Geometry check sheet. Reference: the model listing, model coordinates, mm. A direction names the side the tool comes from. Coordinates: 2 decimals unless noted, no trailing zeros. Order: outer loops, then holes, each group sorted by start corner. A loop starts at its lowest first (then second) coordinate and runs counter-clockwise, first axis right, second up. Notation, with made-up numbers: (82, 27.25) - (135, 27.25) arc R20 cw to (135, 35.25) - close; hole circle Ø7 at (46.5, 37). An arc over 180 degrees is marked (long way). Return JSON: item names as keys, results as strings. Group by question number.
Item 1: Section check C-C on y = 31. Enter the section's corners in (x, z), then the cut area to 3 significant figures.
Item 2: Scan lines: probe 1 along Z at (x, y) = (13.5, 37); probe 2 along Y at (x, z) = (9, -0.5); probe 3 along X at (y, z) = (0.75, -12.5). Record each from-to range of solid material in increasing order.
Item 3: Gauge pin test, flat ends, axial feed: pin 1 (7.5 mm diameter, centred on x = 10.5, y = 15, fed in from -Z); pin 2 (0.6 mm diameter, centred on y = 0.5, z = -24, fed in from -X); pin 3 (2 mm diameter, centred on y = 27.5, z = -10, fed in from -X). Record the tip position at first contact, or that the pin passes through.
Item 4: Section check D-D on x = 13.5. Enter the section's corners in (y, z), then the cut area to 3 significant figures.
Item 5: Section check A-A on x = 24. Enter the section's corners in (y, z).
Item 6: Draft check along Z on faces 5 (the flat face through (25.2, 12.4, -25)), 6 (the cylindrical face through (16, 40.9, -11.4)), 7 (the flat face through (17.9, 2, -9.5)). Enter one of: pulls with the +Z half, pulls with the -Z half, needs draft (parallel to the pull), parting line crosses it, or undercut.
Item 7: Section check B-B on z = -11.5. Enter the section's corners in (x, y), then the cut area to 3 significant figures.
Item 8: Tool access check on faces 1 (the flat face through (11.5, 41, -12)), 2 (the cylindrical face through (7.518, 31.014, -17.871)), 3 (the cylindrical face through (16.56, 1.01, -16.92)), 4 (the flat face through (13, 16, 0)). Record the directions out of +Z, -Z, +X, -X, +Y, -Y that give a thin tool (end or side, any length) a straight path to the whole face; none if there is none.
from build123d import *

# Parameters (mm, degrees)
SKETCH1_W           = 25
SKETCH1_H           = 2
EXTRUDE_THIN1_DEPTH = 25
SKETCH2_R           = 6.0005
CUT_EXTRUDE1_DEPTH  = 36.411862419
BOSS_EXTRUDE1_DEPTH = 32
BOSS_EXTRUDE2_DEPTH = 2
SKETCH7_R           = 3.5
BOSS_EXTRUDE3_DEPTH = 18


with BuildPart() as part:
    # Sketch1 → Extrude-Thin1 (new body)
    with BuildSketch(Plane.XY):
        with Locations((12.5, 1)):
            Rectangle(SKETCH1_W, SKETCH1_H)
    extrude(amount=-EXTRUDE_THIN1_DEPTH)

    # Sketch2 → Cut-Extrude1 (cut, through all)
    with BuildSketch(Plane(origin=(0, 2, 0), x_dir=(1, 0, 0), z_dir=(0, 1, 0))):
        with BuildLine():
            ThreePointArc((3.839745962, 7.5), (3.839745962, 17.5), (12.5, 22.5))
            Line((12.5, 22.5), (12.5, 25))
            Line((12.5, 25), (0, 25))
            Line((0, 25), (0, 7.5))
            Line((0, 7.5), (3.839745962, 7.5))
        make_face()
        with Locations(Location((12.5, 12.5, 0), (0, 0, 270))):
            Circle(SKETCH2_R)
    extrude(amount=-CUT_EXTRUDE1_DEPTH, mode=Mode.SUBTRACT)

    # Sketch4 → Boss-Extrude1 (add)
    with BuildSketch(Plane.XZ):
        Polygon((0, 0), (0, 2), (27, 2), (27, -25), (25, -25), (25, 0), align=None)
    extrude(amount=-BOSS_EXTRUDE1_DEPTH)

    # Sketch6 → Boss-Extrude2 (add)
    with BuildSketch(Plane(origin=(0, 32, 0), x_dir=(1, 0, 0), z_dir=(0, 1, 0))):
        with BuildLine():
            Line((0, 0), (25, 0))
            Line((25, 0), (25, 25))
            ThreePointArc((25, 25), (7.32233047, 17.67766953), (0, 0))
        make_face()
    extrude(amount=-BOSS_EXTRUDE2_DEPTH)

    # Sketch7 → Boss-Extrude3 (add)
    with BuildSketch(Plane(origin=(0, 32, 0), x_dir=(1, 0, 0), z_dir=(0, 1, 0))):
        with Locations(Location((13.5, 11.5, 0), (0, 0, 90))):
            Circle(SKETCH7_R)
        with BuildLine():
            Line((11.5, 13), (11.5, 10))
            ThreePointArc((11.5, 10), (16, 11.5), (11.5, 13))
        make_face(mode=Mode.SUBTRACT)
    extrude(amount=BOSS_EXTRUDE3_DEPTH)


solid = part.part
Computed:
{
 "1": {"outline": "(0, 0) arc R25 ccw to (25, -25) - (27, -25) - (27, 2) - (0, 2) - close", "area": "595 mm²"},
 "2": {"probe 1": "z = -15 to -14, -9 to -8", "probe 2": "y = 0 to 2, 30 to 32", "probe 3": "x = 2.5 to 6.5, 18.5 to 27"},
 "3": {"pin 1": "stops at z = 0", "pin 2": "stops at x = 12.5", "pin 3": "stops at x = 25"},
 "4": {"outline": "(0, -25) - (2, -25) - (2, -18.42) - (0, -18.42) - close; (0, -6.58) - (2, -6.58) - (2, 0) - (30, 0) - (30, -22.2) - (32, -22.2) - (32, -15) - (50, -15) - (50, -14) - (32, -14) - (32, -9) - (50, -9) - (50, -8) - (32, -8) - (32, 2) - (0, 2) - close", "area": "171 mm²"},
 "5": {"outline": "(0, -25) - (2, -25) - (2, 0) - (30, 0) - (30, -24.98) - (32, -24.98) - (32, 2) - (0, 2) - close"},
 "6": {"face 5": "pulls with the -Z half", "face 6": "undercut", "face 7": "needs draft"},
 "7": {"outline": "(2.55, 0) - (6.58, 0) - (6.58, 2) - (2.55, 2) - close; (2.8, 30) - (25, 30) - (25, 2) - (18.42, 2) - (18.42, 0) - (27, 0) - (27, 32) - (17, 32) - (17, 50) - (16, 50) - (16, 32) - (11.5, 32) - (11.5, 50) - (10, 50) - (10, 32) - (2.8, 32) - close", "area": "175 mm²"},
 "8": {"face 1": "+Y", "face 2": "-Z, -X, +Y", "face 3": "-Y", "face 4": "-Z, -X"}
}
